Check sheet for the modelled part. Datum: model origin and axes. Units: mm. A direction names the side the tool comes from. Coordinates: 2 decimals unless noted, no trailing zeros. Loops run counter-clockwise (first coordinate to the right, second up) from the corner with the lowest first, then second, coordinate; pieces in that order, holes last. Notation, with made-up numbers: (-12.75, -26) - (13.25, -26) arc R6 cw to (13.25, -16) - close; hole circle Ø3 at (76.25, 24). An arc over 180 degrees is marked (long way). Use a Markdown table: item, result. Add a question column.
1) Tool access check on faces 4 (the flat face through (-7.75, 21, 33)), 5 (the flat face through (10, -19, 31.2)), 6 (the flat face through (-7.75, -21, 33)), 7 (the flat face through (7.75, -21, 1)), 8 (the flat face through (11, 20, 24)). Record the directions out of +Z, -Z, +X, -X, +Y, -Y that give a thin tool (end or side, any length) a straight path to the whole face; none if there is none.
2) Draft check along Y on faces 1 (the flat face through (0, 23.25, 17)), 2 (the flat face through (0, -6.25, 2)), 3 (the flat face through (0, -23.25, 17)). Enter one of: pulls with the +Y half, pulls with the -Y half, needs draft (parallel to the pull), parting line crosses it, or undercut.
3) Sectioned sample at B-B, the plane y = 12. Enter the section's corners in (x, z), then the cut area to 4 significant figures.
4) Sectioned sample at C-C, the plane z = 32. Enter the section's corners in (x, y), then the cut area to 3 significant figures.
5) Thickness scan on line 1 (X direction, y = -20, z = 8.75); line 2 (Y direction, x = -11, z = 4.75). Record the ranges inside material, lowest first.
6) Sectioned sample at D-D, the plane z = 20. Enter the section's corners in (x, y), then the cut area to 3 significant figures.
7) Go/stop test with flat-tipped pins: P1, Ø4, axis at x = -11, y = 20, coming from the +Z side; P2, Ø1.4, axis at x = 12, z = 32.5, coming from the +Y side; P3, Ø2, axis at x = 11.5, y = 20, coming from the -Z side. Record where each tip stops, or that it passes through.
8) Sectioned sample at A-A, the plane x = 0. Enter the section's corners in (y, z), then the cut area to 3 significant figures.
from build123d import *

# Parameters (mm, degrees)
SKETCH1_W           = 28.5
SKETCH1_H           = 46.5
BOSS_EXTRUDE1_DEPTH = 34
SKETCH2_R           = 10.25
CUT_EXTRUDE1_DEPTH  = 35
SKETCH3_R           = 1.25
CUT_EXTRUDE2_DEPTH  = 10
CUT_EXTRUDE3_DEPTH  = 0.5
CUT_EXTRUDE4_DEPTH  = 2.8
SKETCH6_W           = 28.5
SKETCH6_H           = 10
CUT_EXTRUDE5_DEPTH  = 4
CHAMFER1_SIZE       = 1
CHAMFER2_SIZE       = 0.5
CHAMFER3_SIZE       = 0.5


with BuildPart() as part:
    # Sketch1 → Boss-Extrude1 (new body)
    with BuildSketch(Plane.XY):
        Rectangle(SKETCH1_W, SKETCH1_H)
    extrude(amount=BOSS_EXTRUDE1_DEPTH)

    # Sketch2 → Cut-Extrude1 (cut, through all)
    with BuildSketch(Plane.XY.offset(34)):
        with Locations((0, 12)):
            Circle(SKETCH2_R)
    extrude(amount=-CUT_EXTRUDE1_DEPTH, mode=Mode.SUBTRACT)

    # Sketch3 → Cut-Extrude2 (cut)
    with BuildSketch(Plane.XY.offset(34)):
        with Locations((-11, 20)):
            Circle(SKETCH3_R)
        with Locations((11, 20)):
            Circle(SKETCH3_R)
        with Locations((11, -20)):
            Circle(SKETCH3_R)
        with Locations((-11, -20)):
            Circle(SKETCH3_R)
    cut_extrude2 = extrude(amount=-CUT_EXTRUDE2_DEPTH, mode=Mode.SUBTRACT)

    # Sketch4 → Cut-Extrude3 (cut)
    with BuildSketch(Plane.XY.offset(34)):
        with BuildLine():
            Line((-5, -20.75), (5, -20.75))
            ThreePointArc((5, -20.75), (5.707106781, -20.457106781), (6, -19.75))
            Line((6, -19.75), (6, -14.75))
            ThreePointArc((6, -14.75), (5.707106781, -14.042893219), (5, -13.75))
            Line((5, -13.75), (-5, -13.75))
            ThreePointArc((-5, -13.75), (-5.707106781, -14.042893219), (-6, -14.75))
            Line((-6, -14.75), (-6, -19.75))
            ThreePointArc((-6, -19.75), (-5.707106781, -20.457106781), (-5, -20.75))
        make_face()
    extrude(amount=-CUT_EXTRUDE3_DEPTH, mode=Mode.SUBTRACT)

    # Sketch5 → Cut-Extrude4 (cut)
    with BuildSketch(Plane.XY.offset(34)):
        with BuildLine():
            Line((-7.75, 23.25), (-11, 23.25))
            ThreePointArc((-11, 23.25), (-8.701902961, 22.298097039), (-7.75, 20))
            Line((-7.75, 20), (-7.75, 23.25))
        make_face()
        with BuildLine():
            Line((-11, 23.25), (-14.25, 23.25))
            Line((-14.25, 23.25), (-14.25, 20))
            ThreePointArc((-14.25, 20), (-13.298097039, 22.298097039), (-11, 23.25))
        make_face()
        with BuildLine():
            ThreePointArc((-11, 16.75), (-13.298097039, 17.701902961), (-14.25, 20))
            Line((-14.25, 20), (-14.25, 16.75))
            Line((-14.25, 16.75), (-11, 16.75))
        make_face()
        with BuildLine():
            Line((-12.25, 20), (-14.25, 20))
            ThreePointArc((-14.25, 20), (-13.298097039, 17.701902961), (-11, 16.75))
            Line((-11, 16.75), (-11, 18.75))
            ThreePointArc((-11, 18.75), (-11.883883476, 19.116116524), (-12.25, 20))
        make_face()
        with BuildLine():
            ThreePointArc((-11, 16.75), (-8.701902961, 17.701902961), (-7.75, 20))
            Line((-7.75, 20), (-9.75, 20))
            ThreePointArc((-9.75, 20), (-10.116116524, 19.116116524), (-11, 18.75))
            Line((-11, 18.75), (-11, 16.75))
        make_face()
        with BuildLine():
            ThreePointArc((-7.75, 20), (-8.701902961, 22.298097039), (-11, 23.25))
            ThreePointArc((-11, 23.25), (-13.298097039, 22.298097039), (-14.25, 20))
            Line((-14.25, 20), (-12.25, 20))
            ThreePointArc((-12.25, 20), (-11, 21.25), (-9.75, 20))
            Line((-9.75, 20), (-7.75, 20))
        make_face()
        with BuildLine():
            Line((11, 23.25), (7.75, 23.25))
            Line((7.75, 23.25), (7.75, 20))
            ThreePointArc((7.75, 20), (8.701902961, 22.298097039), (11, 23.25))
        make_face()
        with BuildLine():
            Line((14.25, 23.25), (11, 23.25))
            ThreePointArc((11, 23.25), (13.298097039, 22.298097039), (14.25, 20))
            Line((14.25, 20), (14.25, 23.25))
        make_face()
        with BuildLine():
            ThreePointArc((14.25, 20), (13.298097039, 17.701902961), (11, 16.75))
            Line((11, 16.75), (14.25, 16.75))
            Line((14.25, 16.75), (14.25, 20))
        make_face()
        with BuildLine():
            Line((9.75, 20), (7.75, 20))
            ThreePointArc((7.75, 20), (8.701902961, 17.701902961), (11, 16.75))
            Line((11, 16.75), (11, 18.75))
            ThreePointArc((11, 18.75), (10.116116524, 19.116116524), (9.75, 20))
        make_face()
        with BuildLine():
            Line((11, 18.75), (11, 16.75))
            ThreePointArc((11, 16.75), (13.298097039, 17.701902961), (14.25, 20))
            Line((14.25, 20), (12.25, 20))
            ThreePointArc((12.25, 20), (11.883883476, 19.116116524), (11, 18.75))
        make_face()
        with BuildLine():
            ThreePointArc((11, 23.25), (8.701902961, 22.298097039), (7.75, 20))
            Line((7.75, 20), (9.75, 20))
            ThreePointArc((9.75, 20), (11, 21.25), (12.25, 20))
            Line((12.25, 20), (14.25, 20))
            ThreePointArc((14.25, 20), (13.298097039, 22.298097039), (11, 23.25))
        make_face()
        with BuildLine():
            ThreePointArc((-11, -16.75), (-13.298097039, -17.701902961), (-14.25, -20))
            Line((-14.25, -20), (-12.25, -20))
            ThreePointArc((-12.25, -20), (-11.883883476, -19.116116524), (-11, -18.75))
            Line((-11, -18.75), (-11, -16.75))
        make_face()
        with BuildLine():
            ThreePointArc((-7.75, -20), (-8.701902961, -17.701902961), (-11, -16.75))
            Line((-11, -16.75), (-11, -18.75))
            ThreePointArc((-11, -18.75), (-10.116116524, -19.116116524), (-9.75, -20))
            Line((-9.75, -20), (-7.75, -20))
        make_face()
        with BuildLine():
            Line((-12.25, -20), (-14.25, -20))
            ThreePointArc((-14.25, -20), (-13.298097039, -22.298097039), (-11, -23.25))
            ThreePointArc((-11, -23.25), (-8.701902961, -22.298097039), (-7.75, -20))
            Line((-7.75, -20), (-9.75, -20))
            ThreePointArc((-9.75, -20), (-11, -21.25), (-12.25, -20))
        make_face()
        with BuildLine():
            Line((-11, -16.75), (-14.25, -16.75))
            Line((-14.25, -16.75), (-14.25, -20))
            ThreePointArc((-14.25, -20), (-13.298097039, -17.701902961), (-11, -16.75))
        make_face()
        with BuildLine():
            ThreePointArc((-11, -23.25), (-13.298097039, -22.298097039), (-14.25, -20))
            Line((-14.25, -20), (-14.25, -23.25))
            Line((-14.25, -23.25), (-11, -23.25))
        make_face()
        with BuildLine():
            ThreePointArc((-7.75, -20), (-8.701902961, -22.298097039), (-11, -23.25))
            Line((-11, -23.25), (-7.75, -23.25))
            Line((-7.75, -23.25), (-7.75, -20))
        make_face()
        with BuildLine():
            Line((7.75, -20), (7.75, -23.25))
            Line((7.75, -23.25), (11, -23.25))
            ThreePointArc((11, -23.25), (8.701902961, -22.298097039), (7.75, -20))
        make_face()
        with BuildLine():
            ThreePointArc((11, -23.25), (13.298097039, -22.298097039), (14.25, -20))
            Line((14.25, -20), (12.25, -20))
            ThreePointArc((12.25, -20), (11, -21.25), (9.75, -20))
            Line((9.75, -20), (7.75, -20))
            ThreePointArc((7.75, -20), (8.701902961, -22.298097039), (11, -23.25))
        make_face()
        with BuildLine():
            Line((14.25, -23.25), (14.25, -20))
            ThreePointArc((14.25, -20), (13.298097039, -22.298097039), (11, -23.25))
            Line((11, -23.25), (14.25, -23.25))
        make_face()
        with BuildLine():
            ThreePointArc((14.25, -20), (13.298097039, -17.701902961), (11, -16.75))
            Line((11, -16.75), (11, -18.75))
            ThreePointArc((11, -18.75), (11.883883476, -19.116116524), (12.25, -20))
            Line((12.25, -20), (14.25, -20))
        make_face()
        with BuildLine():
            Line((11, -18.75), (11, -16.75))
            ThreePointArc((11, -16.75), (8.701902961, -17.701902961), (7.75, -20))
            Line((7.75, -20), (9.75, -20))
            ThreePointArc((9.75, -20), (10.116116524, -19.116116524), (11, -18.75))
        make_face()
        with BuildLine():
            Line((14.25, -20), (14.25, -16.75))
            Line((14.25, -16.75), (11, -16.75))
            ThreePointArc((11, -16.75), (13.298097039, -17.701902961), (14.25, -20))
        make_face()
    cut_extrude4 = extrude(amount=-CUT_EXTRUDE4_DEPTH, mode=Mode.SUBTRACT)

    # Mirror1: Cut-Extrude4 across plane
    add(cut_extrude4.mirror(Plane.XY.offset(17)), mode=Mode.SUBTRACT)

    # Mirror2: Cut-Extrude2 across plane
    add(cut_extrude2.mirror(Plane.XY.offset(17)), mode=Mode.SUBTRACT)

    # Sketch6 → Cut-Extrude5 (cut)
    with BuildSketch(Plane(origin=(0, 0, 0), x_dir=(-1, 0, 0), z_dir=(0, 0, -1))):
        with Locations((0, -1.25)):
            Rectangle(SKETCH6_W, SKETCH6_H)
    extrude(amount=-CUT_EXTRUDE5_DEPTH, mode=Mode.SUBTRACT)

    # Chamfer1
    chamfer1_edges = [part.edges().sort_by_distance(p)[0] for p in [
        (14.25, -23.25, 17),
        (-14.25, -23.25, 17),
        (-14.25, 23.25, 17),
        (14.25, 23.25, 17),
    ]]
    chamfer(chamfer1_edges, length=CHAMFER1_SIZE)

    # Chamfer2
    chamfer2_edges = [part.edges().sort_by_distance(p)[0] for p in [
        (-14.25, 10.25, 0),
        (0, 23.25, 0),
        (7.75, 23.25, 1.4),
        (14.25, 16.75, 1.4),
        (14.25, 19.5, 2.8),
        (-14.25, 16.75, 1.4),
        (-10.5, 23.25, 2.8),
        (14.25, 10.25, 0),
        (-14.25, 19.5, 2.8),
        (-13.75, 22.75, 2.8),
        (10.5, 23.25, 2.8),
        (13.75, 22.75, 2.8),
    ]]
    chamfer(chamfer2_edges, length=CHAMFER2_SIZE)

    # Chamfer3
    chamfer3_edges = [part.edges().sort_by_distance(p)[0] for p in [
        (-9.916381265, 3.75, 0),
        (9.916381265, 3.75, 0),
        (-14.25, -11.5, 0),
        (-14.25, -19.5, 2.8),
        (-13.75, -22.75, 31.2),
        (-13.75, -22.75, 2.8),
        (-10.5, -23.25, 2.8),
        (-7.75, -23.25, 1.4),
        (14.25, -11.5, 0),
        (14.25, -16.75, 1.4),
        (0, -23.25, 0),
        (7.75, -23.25, 1.4),
        (10.5, -23.25, 2.8),
        (14.25, -19.5, 2.8),
        (13.75, -22.75, 31.2),
        (13.75, -22.75, 2.8),
        (-14.25, -19.5, 31.2),
        (-10.5, -23.25, 31.2),
        (-7.75, -23.25, 32.6),
        (0, -23.25, 34),
        (7.75, -23.25, 32.6),
        (14.25, -19.5, 31.2),
        (10.5, -23.25, 31.2),
        (14.25, 0, 34),
        (14.25, 16.75, 32.6),
        (14.25, 19.5, 31.2),
        (13.75, 22.75, 31.2),
        (10.5, 23.25, 31.2),
        (7.75, 23.25, 32.6),
        (0, 23.25, 34),
        (-7.75, 23.25, 32.6),
        (-14.25, 0, 34),
        (-14.25, 16.75, 32.6),
        (-14.25, 19.5, 31.2),
        (-13.75, 22.75, 31.2),
        (-10.5, 23.25, 31.2),
    ]]
    chamfer(chamfer3_edges, length=CHAMFER3_SIZE)


solid = part.part
Solved:
| question | item | result |
|---|---|---|
| 1 | face 4 | +Z, -X, +Y |
| 1 | face 5 | +Z, +X, -Y |
| 1 | face 6 | +Z, -X, -Y |
| 1 | face 7 | -Z, +X, -Y |
| 1 | face 8 | +Z |
| 2 | face 1 | pulls with the +Y half |
| 2 | face 2 | undercut |
| 2 | face 3 | pulls with the -Y half |
| 3 | outline | (-14.25, 0.5) - (-13.75, 0) - (-10.25, 0) - (-10.25, 34) - (-13.75, 34) - (-14.25, 33.5) - close; (10.25, 0) - (13.75, 0) - (14.25, 0.5) - (14.25, 33.5) - (13.75, 34) - (10.25, 34) - close |
| 3 | area | 271.5 mm2 |
| 4 | outline | (-14.25, -16.75) - (-11, -16.75) arc R3.25 cw to (-7.75, -20) - (-7.75, -22.75) - (-7.25, -23.25) - (7.25, -23.25) - (7.75, -22.75) - (7.75, -20) arc R3.25 cw to (11, -16.75) - (14.25, -16.75) - (14.25, 16.25) - (13.75, 16.75) - (11, 16.75) arc R3.25 cw to (7.75, 20) - (7.75, 22.75) - (7.25, 23.25) - (-7.25, 23.25) - (-7.75, 22.75) - (-7.75, 20) arc R3.25 cw to (-11, 16.75) - (-13.75, 16.75) - (-14.25, 16.25) - close; hole circle Ø20.5 at (0, 12) |
| 4 | area | 835 mm2 |
| 5 | line 1 | x = -14.25 to -12.25, -9.75 to 9.75, 12.25 to 14.25 |
| 5 | line 2 | y = -23.25 to -21.25, -18.75 to 18.75, 21.25 to 23.25 |
| 6 | outline | (-14.25, -22.25) - (-13.25, -23.25) - (13.25, -23.25) - (14.25, -22.25) - (14.25, 22.25) - (13.25, 23.25) - (-13.25, 23.25) - (-14.25, 22.25) - close; hole circle Ø20.5 at (0, 12) |
| 6 | area | 993 mm2 |
| 7 | P1 | stops at z = 31.2 |
| 7 | P2 | stops at y = 16.75 |
| 7 | P3 | stops at z = 2.8 |
| 8 | outline | (-23.25, 0.5) - (-22.75, 0) - (-6.25, 0) - (-6.25, 4) - (1.75, 4) - (1.75, 34) - (-13.75, 34) - (-13.75, 33.5) - (-20.75, 33.5) - (-20.75, 34) - (-22.75, 34) - (-23.25, 33.5) - close; (22.25, 0) - (22.75, 0) - (23.25, 0.5) - (23.25, 33.5) - (22.75, 34) - (22.25, 34) - close |
| 8 | area | 848 mm2 |
